For this review, take the finished solid that the model builds, in its own axes (mm). Give positions to 0.01 mm unless a question says otherwise; leave off trailing zeros. Loops run counter-clockwise (first coordinate to the right, second up) from the corner with the lowest first, then second, coordinate; pieces in that order, holes last. Notation, with made-up numbers: (49, 75) - (104, 75) arc R22 ccw to (104, 86) - close; hole circle Ø4 at (57.5, 84.5). An arc over 180 degrees is marked (long way). Answer as CSV lines item,"result".
from build123d import *

# Parameters (mm, degrees)
F0_R     = 1.7526
F0_R_2   = 2.5527
F0_R_3   = 11.1125
F1_DEPTH = 3.175


with BuildPart() as f1:
    # F0 (on Front) → F1 (new body)
    with BuildSketch(Plane.XZ):
        with BuildLine():
            Line((-46.642908, 5.291286), (-45.682848, 5.593446))
            ThreePointArc((-45.682848, 5.593446), (-46.169528, 5.463494), (-46.642908, 5.291286))
        make_face()
        with BuildLine():
            Line((-5.71905, 18.171268), (-45.682848, 5.593446))
            Line((-45.682848, 5.593446), (-46.642908, 5.291286))
            ThreePointArc((-46.642908, 5.291286), (-50.1777, 0), (-46.642908, -5.291286))
            Line((-46.642908, -5.291286), (-45.682848, -5.593446))
            Line((-45.682848, -5.593446), (-5.71905, -18.171268))
            ThreePointArc((-5.71905, -18.171268), (0, -19.05), (5.71905, -18.171268))
            Line((5.71905, -18.171268), (45.682848, -5.593446))
            Line((45.682848, -5.593446), (46.642908, -5.291286))
            ThreePointArc((46.642908, -5.291286), (50.1777, 0), (46.642908, 5.291286))
            Line((46.642908, 5.291286), (45.682848, 5.593446))
            Line((45.682848, 5.593446), (5.71905, 18.171268))
            ThreePointArc((5.71905, 18.171268), (0, 19.05), (-5.71905, 18.171268))
        make_face()
        with Locations((-10.960097, -10.960097)):
            Circle(F0_R, mode=Mode.SUBTRACT)
        with Locations((-44.45, 0)):
            Circle(F0_R_2, mode=Mode.SUBTRACT)
        with Locations((10.960097, -10.960097)):
            Circle(F0_R, mode=Mode.SUBTRACT)
        Circle(F0_R_3, mode=Mode.SUBTRACT)
        with Locations((44.45, 0)):
            Circle(F0_R_2, mode=Mode.SUBTRACT)
        with Locations((-10.960097, 10.960097)):
            Circle(F0_R, mode=Mode.SUBTRACT)
        with Locations((10.960097, 10.960097)):
            Circle(F0_R, mode=Mode.SUBTRACT)
        with BuildLine():
            Line((-45.682848, -5.593446), (-46.642908, -5.291286))
            ThreePointArc((-46.642908, -5.291286), (-46.169528, -5.463494), (-45.682848, -5.593446))
        make_face()
        with BuildLine():
            ThreePointArc((46.642908, 5.291286), (46.169528, 5.463494), (45.682848, 5.593446))
            Line((45.682848, 5.593446), (46.642908, 5.291286))
        make_face()
        with BuildLine():
            ThreePointArc((45.682848, -5.593446), (46.169528, -5.463494), (46.642908, -5.291286))
            Line((46.642908, -5.291286), (45.682848, -5.593446))
        make_face()
    extrude(amount=F1_DEPTH)


solid = f1.part
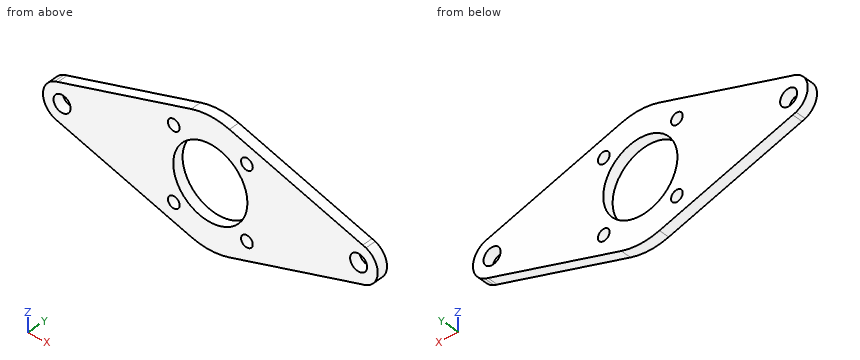
1) Consider section C-C on x = -44.45. Write out the cut boundary in (y, z) (3 decimals), and give its area (3 significant figures).
From the geometry:
outline,"(-3.175, -5.981) - (0, -5.981) - (0, -2.553) - (-3.175, -2.553) - close; (-3.175, 2.553) - (0, 2.553) - (0, 5.981) - (-3.175, 5.981) - close"
area,"21.8 mm^2"
2) Consider section B-B on z = 0. Write out the cut boundary in (x, y) (1 decimal).
From the geometry:
outline,"(-50.2, -3.2) - (-47, -3.2) - (-47, 0) - (-50.2, 0) - close; (-41.9, -3.2) - (-11.1, -3.2) - (-11.1, 0) - (-41.9, 0) - close; (11.1, -3.2) - (41.9, -3.2) - (41.9, 0) - (11.1, 0) - close; (47, -3.2) - (50.2, -3.2) - (50.2, 0) - (47, 0) - close"
3) Consider section D-D on x = 33.5. Write out the cut boundary in (y, z) (3 decimals).
From the geometry:
outline,"(-3.175, -9.428) - (0, -9.428) - (0, 9.428) - (-3.175, 9.428) - close"
4) Insertion check: P1, Ø1, axis at x = -33.5, y = -1.5, coming from the +Z side; P2, Ø1.5, axis at y = -2.5, z = 2, coming from the -X side. Each pin has a flat end and moves straight along its axis. Give the tip position at first contact, or say it passes through.
From the geometry:
P1,"stops at z = 9.59"
P2,"stops at x = -50.04"
5) Wall thickness on line 1 (Z direction, x = 0, y = -1.45); line 2 (Z direction, x = -5.5, y = -2.2); line 3 (X direction, y = -2, z = -4): over which ranges is each line inside the solid? List them lowest first. Write a range as from..to.
From the geometry:
line 1,"z = -19.05..-11.11, 11.11..19.05"
line 2,"z = -18.24..-9.66, 9.66..18.24"
line 3,"x = -48.55..-10.37, 10.37..48.55"
